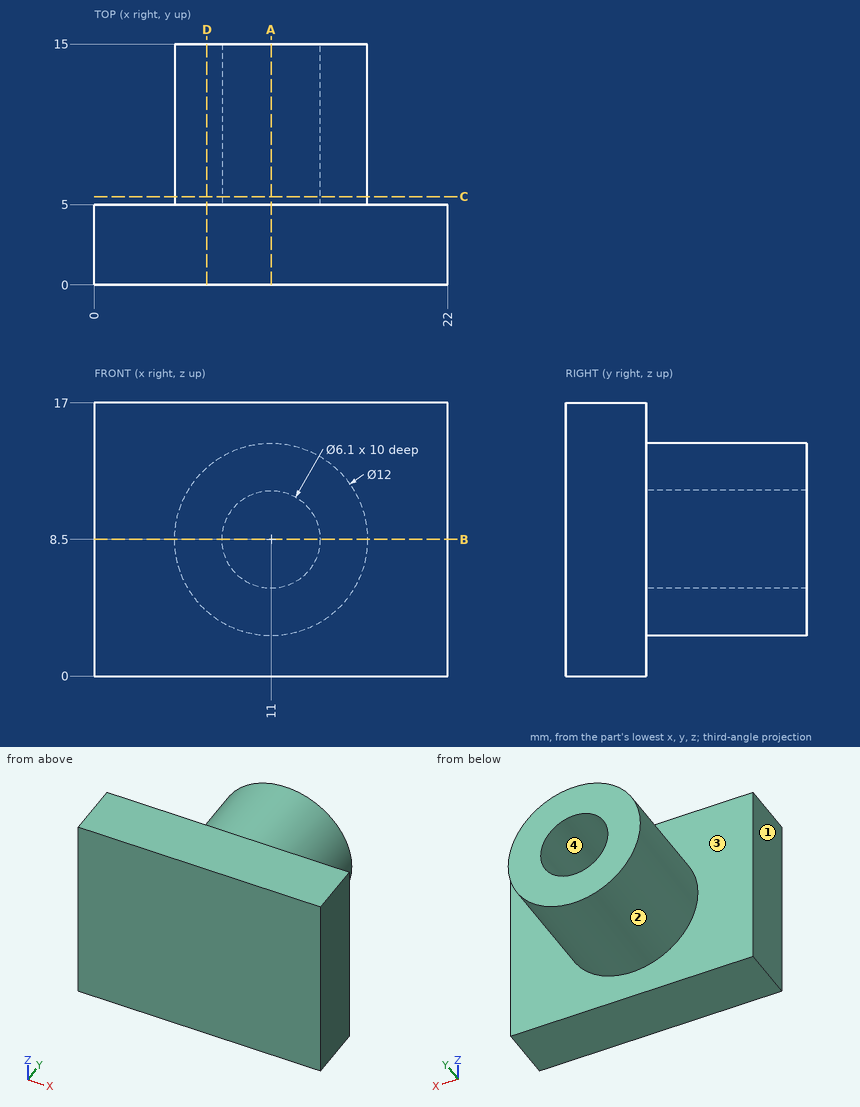
Design review of the part shown in the three views and the two pictorial views. Dimensions are in mm from the part's minimum x, y and z. Give positions to 0.01 mm unless a question says otherwise; leave off trailing zeros. Write each loop counter-clockwise with the first axis right and the second up, starting at its lowest first coordinate (ties: lowest second). Pieces come first, ordered by that corner, then holes. Notation, with made-up numbers: (-35, 2.25) - (6, 2.25) arc R31 ccw to (6, 27.25) - close; hole circle Ø6 at (8.25, -7). An arc over 180 degrees is marked (long way). Return JSON: item names as keys, results as strings. Group by question number.
(1) Mouldability with a two-part tool opening along X and no side actions: class the marked faces 1, 2, 3 and 4 as +X half, -X half, draft (parallel to the pull), parting line (faces both ways), or undercut.
(2) We need section A-A, the plane x = 11. Give the boundary of the cut face in (y, z), then the cut area to 3 significant figures.
(3) We need section B-B, the plane z = 8.5. Give the boundary of the cut face in (x, y).
(4) We need section C-C, the plane y = 5.5. Give the boundary of the cut face in (x, z), then the cut area to 3 significant figures.
(5) We need section D-D, the plane x = 7. Give the boundary of the cut face in (y, z).
(6) To check wall thickness, follow probe 1 along Z at (x, y) = (11, 10.75); probe 2 along X at (y, z) = (8, 8.5); probe 3 along Y at (x, z) = (9.25, 7.25). State the ranges of each line that lie inside material, in increasing order.
(7) Insertion check: pin 1 (5 mm diameter, centred on x = 5, z = 2, fed in from +Y); pin 2 (5 mm diameter, centred on y = 10.5, z = 12, fed in from +X); pin 3 (3 mm diameter, centred on x = 19.5, y = 9, fed in from +Z). Each pin has a flat end and moves straight along its axis. Give the tip position at first contact, or say it passes through.
Reported:
{
 "1": {"face 1": "-X half", "face 2": "parting line", "face 3": "draft", "face 4": "undercut"},
 "2": {"outline": "(0, 0) - (5, 0) - (5, 2.5) - (15, 2.5) - (15, 5.45) - (5, 5.45) - (5, 11.55) - (15, 11.55) - (15, 14.5) - (5, 14.5) - (5, 17) - (0, 17) - close", "area": "144 mm2"},
 "3": {"outline": "(0, 0) - (22, 0) - (22, 5) - (17, 5) - (17, 15) - (14.05, 15) - (14.05, 5) - (7.95, 5) - (7.95, 15) - (5, 15) - (5, 5) - (0, 5) - close"},
 "4": {"outline": "circle Ø12 at (11, 8.5); hole circle Ø6.1 at (11, 8.5)", "area": "83.9 mm2"},
 "5": {"outline": "(0, 0) - (5, 0) - (5, 4.03) - (15, 4.03) - (15, 12.97) - (5, 12.97) - (5, 17) - (0, 17) - close"},
 "6": {"probe 1": "z = 2.5 to 5.45, 11.55 to 14.5", "probe 2": "x = 5 to 7.95, 14.05 to 17", "probe 3": "y = 0 to 5"},
 "7": {"pin 1": "stops at y = 5", "pin 2": "stops at x = 16.92", "pin 3": "passes through"}
}
